from build123d import *

# Parameters (mm, degrees)
BOSS_EXTRUDE1_DEPTH = 10.16
FILLET1_R           = 19.05
SKETCH2_W           = 120.284747719
SKETCH2_H           = 20.32
SKETCH2_W_2         = 102.891608588
CUT_EXTRUDE1_DEPTH  = 12.7


with BuildPart() as part:
    # Sketch1 → Boss-Extrude1 (new body)
    with BuildSketch(Plane.XY):
        Polygon((-288.275887252, 0), (-215.032557346, 1054.1), (215.032557346, 1054.1), (288.275887252, 0), (596.950713016, 0), (596.950713016, 20.32), (457.769290722, 178.8375841), (368.537470958, 1463.04), (215.892500906, 1463.04), (-205.715298803, 1463.040000035), (-647.718210796, 1463.04), (-647.718210796, 0), align=None)
        Polygon((-609.618210796, 127), (-609.618210796, 461.510956689), (-365.626284392, 127), align=None, mode=Mode.SUBTRACT)
        Polygon((-609.618210796, 592.582701044), (-609.618210796, 907.626666667), (-314.736774564, 907.626666667), align=None, mode=Mode.SUBTRACT)
        Polygon((-282.735998162, 867.476761947), (-304.419486117, 555.413333333), (-574.827649063, 555.413333333), align=None, mode=Mode.SUBTRACT)
        Polygon((-307.949285149, 504.613333333), (-331.453012037, 166.353473425), (-578.179384354, 504.613333333), align=None, mode=Mode.SUBTRACT)
        Polygon((-609.618210796, 958.426666667), (-609.618210796, 1288.067621407), (-310.704175954, 958.426666667), align=None, mode=Mode.SUBTRACT)
        Polygon((-575.330448642, 1325.88), (-250.884200804, 1325.88), (-273.976047339, 993.547820907), align=None, mode=Mode.SUBTRACT)
        Polygon((19.05, 1104.9), (19.05, 1368.504716774), (182.716004616, 1104.9), align=None, mode=Mode.SUBTRACT)
        Polygon((41.473134849, 1404.62), (184.313325179, 1404.62), (202.313466912, 1145.566384812), align=None, mode=Mode.SUBTRACT)
        Polygon((-184.313325179, 1404.62), (-41.473134849, 1404.62), (-202.313466912, 1145.566384812), align=None, mode=Mode.SUBTRACT)
        Polygon((-19.05, 1368.504716774), (-19.05, 1104.9), (-182.716004616, 1104.9), align=None, mode=Mode.SUBTRACT)
    extrude(amount=BOSS_EXTRUDE1_DEPTH)

    # Fillet1
    fillet1_edges = [part.edges().sort_by_distance(p)[0] for p in [
        (19.05, 1368.504716774, 5.08),
        (19.05, 1104.9, 5.08),
        (182.716004616, 1104.9, 5.08),
        (-250.884200804, 1325.88, 5.08),
        (-575.330448642, 1325.88, 5.08),
        (-273.976047339, 993.547820907, 5.08),
        (-647.718210796, 1463.04, 5.08),
        (368.537470958, 1463.04, 5.08),
        (457.769290722, 178.8375841, 5.08),
        (215.032557346, 1054.1, 5.08),
        (-215.032557346, 1054.1, 5.08),
        (-609.618210796, 1288.067621407, 5.08),
        (-609.618210796, 958.426666667, 5.08),
        (-310.704175954, 958.426666667, 5.08),
        (-609.618210796, 461.510956689, 5.08),
        (-609.618210796, 127, 5.08),
        (-365.626284392, 127, 5.08),
        (-41.473134849, 1404.62, 5.08),
        (-184.313325179, 1404.62, 5.08),
        (-202.313466912, 1145.566384812, 5.08),
        (-182.716004616, 1104.9, 5.08),
        (-19.05, 1104.9, 5.08),
        (-19.05, 1368.504716774, 5.08),
        (184.313325179, 1404.62, 5.08),
        (41.473134849, 1404.62, 5.08),
        (202.313466912, 1145.566384812, 5.08),
        (-578.179384354, 504.613333333, 5.08),
        (-331.453012037, 166.353473425, 5.08),
        (-307.949285149, 504.613333333, 5.08),
        (-609.618210796, 907.626666667, 5.08),
        (-609.618210796, 592.582701044, 5.08),
        (-314.736774564, 907.626666667, 5.08),
        (-574.827649063, 555.413333333, 5.08),
        (-304.419486117, 555.413333333, 5.08),
        (-282.735998162, 867.476761947, 5.08),
    ]]
    fillet(fillet1_edges, radius=FILLET1_R)

    # Sketch2 → Cut-Extrude1 (cut)
    with BuildSketch(Plane.XY.offset(10.16)):
        with Locations((-467.291089218, 10.16)):
            Rectangle(SKETCH2_W, SKETCH2_H)
        with Locations((442.613300134, 10.16)):
            Rectangle(SKETCH2_W_2, SKETCH2_H)
        Polygon((211.92306481, 1373.664189215), (222.040744894, 1374.366931824), (215.881789204, 1463.040000035), (205.715298803, 1463.040000035), align=None)
        Polygon((234.358656272, 1197.020795404), (227.836927701, 1290.916856945), (217.719247617, 1290.214114336), (224.240976188, 1196.318052795), align=None)
        Polygon((246.676567651, 1019.674658983), (240.15668194, 1113.544188093), (230.039001856, 1112.841445484), (236.558887567, 1018.971916374), align=None)
        Polygon((258.99447903, 842.328522563), (252.476436179, 936.171519242), (242.358756095, 935.468776633), (248.876798945, 841.625779953), align=None)
        Polygon((271.312390408, 664.982386142), (264.796190418, 758.798850391), (254.678510334, 758.096107781), (261.194710324, 664.279643533), align=None)
        Polygon((283.630301787, 487.636249721), (277.115944656, 581.426181539), (266.998264572, 580.72343893), (273.512621703, 486.933507112), align=None)
        Polygon((295.948213166, 310.290113301), (289.435698895, 404.053512688), (279.318018811, 403.350770078), (285.830533081, 309.587370692), align=None)
        Polygon((308.266124544, 132.94397688), (301.755453134, 226.680843836), (291.63777305, 225.978101227), (298.14844446, 132.241234271), align=None)
        Polygon((-301.755453134, 226.680843836), (-308.266124544, 132.94397688), (-298.14844446, 132.241234271), (-291.63777305, 225.978101227), align=None)
        Polygon((-289.435698895, 404.053512688), (-295.948213166, 310.290113301), (-285.830533081, 309.587370692), (-279.318018811, 403.350770078), align=None)
        Polygon((-277.115944656, 581.426181539), (-283.630301787, 487.636249721), (-273.512621703, 486.933507112), (-266.998264572, 580.72343893), align=None)
        Polygon((-264.796190418, 758.798850391), (-271.312390408, 664.982386142), (-261.194710324, 664.279643533), (-254.678510334, 758.096107781), align=None)
        Polygon((-252.476436179, 936.171519242), (-258.99447903, 842.328522563), (-248.876798945, 841.625779953), (-242.358756095, 935.468776633), align=None)
        Polygon((-240.15668194, 1113.544188093), (-246.676567651, 1019.674658983), (-236.558887567, 1018.971916374), (-230.039001856, 1112.841445484), align=None)
        Polygon((-227.836927701, 1290.916856945), (-234.358656272, 1197.020795404), (-224.240976188, 1196.318052795), (-217.719247617, 1290.214114336), align=None)
        Polygon((-222.040744894, 1374.366931824), (-211.92306481, 1373.664189215), (-205.715298803, 1463.040000035), (-215.881789204, 1463.040000035), align=None)
    extrude(amount=-CUT_EXTRUDE1_DEPTH, mode=Mode.SUBTRACT)


solid = part.part
The listing builds one solid part. Answer for the finished solid, in the listing's coordinates (mm). A direction names the side the tool comes from. Give positions to 0.01 mm unless a question says otherwise; leave off trailing zeros. Write each loop counter-clockwise with the first axis right and the second up, starting at its lowest first coordinate (ties: lowest second). Pieces come first, ordered by that corner, then holes.
1) Section C-C (y = 1089) is taken. Write down the section's boundary in (x, z).
2) For a pull along X with two mould halves and no side action, classify faces 4 (the face through (-482.756, 287.584, 5.009)), 5 (the face through (414.16, 806.46, 5.01)), 6 (the face through (-259, 952, 10.16)) as pulls with the +X half, pulls with the -X half, needs draft (parallel to the pull), parting line crosses it, or undercut.
3) Section B-B (x = 114) is taken. Write down the section's boundary in (y, z).
4) Given P1, Ø3, axis at x = 106.5, z = 7, coming from the -Y side; P2, Ø5, axis at y = 802, z = 5.5, coming from the +X side; P3, Ø5, axis at x = 430.5, z = 4.5, coming from the -Y side, each flat-ended and moving along its own axis, determine where each tip first touches the part or whether it passes through.
5) Find the intervals of material crossed by L1, parallel to X at y = 329, z = 9.75; L2, parallel to X at y = 335.5, z = 1; L3, parallel to Y at x = -114, z = 8.5, in increasing order.
6) A tool of negligible diameter and unlimited length cuts with its end or side. For faces 1 (the face through (-457.805, 339.581, 5.009)), 2 (the face through (251.766, 525.44, 5.009)), 3 (the face through (-259, 952, 0)), from which of +Z, -Z, +X, -X, +Y, -Y can it reach the whole face along a straight path? Write none if from no direction.
7) Section A-A (y = 438) is taken. Write down the section's boundary in (x, z), and give its area (3 significant figures).
8) Section D-D (z = 4.5) is taken. Count the separate pieces of the cut face and the enclosed holes in it, and give its area (3 significant figures).
Response:
1. outline: (-647.72, 0) - (-609.62, 0) - (-609.62, 10.16) - (-647.72, 10.16) - close; (-429.11, 0) - (-360.53, 0) - (-360.53, 10.16) - (-429.11, 10.16) - close; (-267.34, 0) - (-241.86, 0) - (-241.86, 10.16) - (-267.34, 10.16) - close; (-231.69, 0) - (231.69, 0) - (231.69, 10.16) - (-231.69, 10.16) - close; (241.86, 0) - (394.53, 0) - (394.53, 10.16) - (241.86, 10.16) - close
2. face 4: undercut
2. face 5: pulls with the +X half
2. face 6: needs draft
3. outline: (1054.1, 0) - (1104.9, 0) - (1104.9, 10.16) - (1054.1, 10.16) - close; (1215.58, 0) - (1287.81, 0) - (1287.81, 10.16) - (1215.58, 10.16) - close; (1404.62, 0) - (1463.04, 0) - (1463.04, 10.16) - (1404.62, 10.16) - close
4. P1: stops at y = 1054.1
4. P2: stops at x = 414.64
4. P3: stops at y = 20.32
5. L1: x = -647.72 to -609.62, -512.96 to -450.09, -320.15 to -294.65, -284.48 to -265.42, 265.42 to 284.48, 294.65 to 447.34
5. L2: x = -647.72 to -609.62, -517.71 to -454.83, -319.7 to -294.2, -284.03 to -264.96, 264.96 to 284.03, 294.2 to 446.88
5. L3: y = 1054.1 to 1104.9, 1215.58 to 1287.81, 1404.62 to 1463.04
6. face 1: +Z, -Z
6. face 2: +Z, -Z, -Y
6. face 3: -Z, +X, -X, +Y, -Y
7. outline: (-647.72, 0) - (-529.59, 0) - (-529.59, 10.16) - (-647.72, 10.16) - close; (-312.58, 0) - (-257.84, 0) - (-257.84, 10.16) - (-312.58, 10.16) - close; (257.84, 0) - (439.76, 0) - (439.76, 10.16) - (257.84, 10.16) - close
7. area: 3,600 mm2
8. separate pieces: 1
8. enclosed holes: 24
8. area: 676,000 mm2
